Autodesk Inventor part; units mm, degrees
ref_plane "YZ Plane" through (0, 0, 0) normal (1, 0, 0) x (0, 1, 0)
ref_plane "XZ Plane" through (0, 0, 0) normal (0, 1, 0) x (-1, 0, 0)
ref_plane "XY Plane" through (0, 0, 0) normal (0, 0, 1) x (1, 0, 0)
sketch "Boceto1" plane through (0, 0, 0) normal (0, 0, 1) x (1, 0, 0)
  line L0 (-200, -200) -> (200, -200)
  line L1 (200, -200) -> (200, 200)
  line L2 (200, 200) -> (-200, 200)
  line L3 (-200, 200) -> (-200, -200)
  line L4 (-200, -200) -> (200, 200) construction
  line L5 (200, -200) -> (-200, 200) construction
  line L6 (-197.5, -197.5) -> (197.5, -197.5)
  line L7 (197.5, -197.5) -> (197.5, 197.5)
  line L8 (197.5, 197.5) -> (-197.5, 197.5)
  line L9 (-197.5, 197.5) -> (-197.5, -197.5)
  line L10 (-197.5, -197.5) -> (197.5, 197.5) construction
  line L11 (197.5, -197.5) -> (-197.5, 197.5) construction
  point P0 (0, 0)
  dimension "d0" = 400
  dimension "d1" = 400
  dimension "d2" = 395
  dimension "d3" = 395
extrude "Extrusión1" add sketch "Boceto1" along normal blind 5 contours L9 L8 L7 L6
extrude "Extrusión2" add sketch "Boceto1" along normal blind 400
properties part number "BOX"
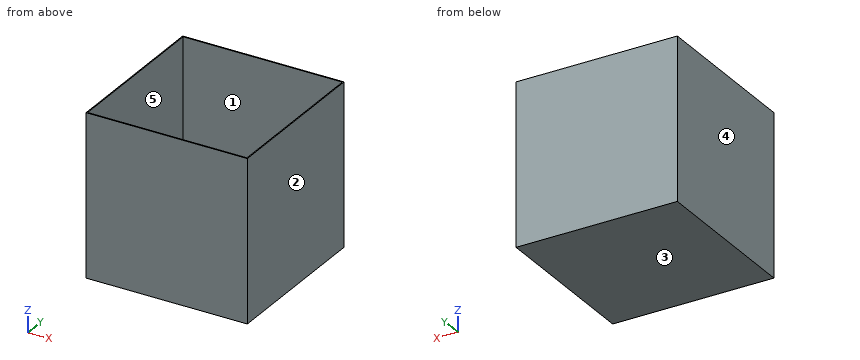
Work out the finished part from the listing and answer in its coordinate system (mm). Face numbers are marked on the shaded views. A direction names the side the tool comes from. Round coordinates to 2 decimals unless told otherwise and drop trailing zeros. Loops run counter-clockwise (first coordinate to the right, second up) from the corner with the lowest first, then second, coordinate; pieces in that order, holes last.
(1) This flat-tipped pin is pushed along its axis until it touches: P1, Ø4, axis at x = 49.5, y = 125.5, coming from the +Z side. Where does it stop, or does it pass through?
Computed values:
P1: stops at z = 5
(2) The part is cut by section B-B, the plane x = 53.5. Give the vertices of the cut face in (y, z).
Computed values:
outline: (-200, 0) - (200, 0) - (200, 400) - (197.5, 400) - (197.5, 5) - (-197.5, 5) - (-197.5, 400) - (-200, 400) - close
(3) For the marked faces 4 and 5, determine the directions among +Z, -Z, +X, -X, +Y, -Y from which every point of the face is accessible in a straight line to the end or side of a thin tool.
Computed values:
face 4: +Z, -Z, -X, +Y, -Y
face 5: +Z
(4) Find the intervals of material crossed by L1, parallel to X at y = 45.5, z = 270; L2, parallel to Z at x = -82, y = 148.5, in increasing order.
Computed values:
L1: x = -200 to -197.5, 197.5 to 200
L2: z = 0 to 5
(5) The mould has two halves that part along X. Classify the marked faces 1, 2 and 3: pulls with the +X half, pulls with the -X half, needs draft (parallel to the pull), parting line crosses it, or undercut.
Computed values:
face 1: undercut
face 2: pulls with the +X half
face 3: needs draft
(6) The part is cut by section A-A, the plane z = 233.5. Give the vertices of the cut face in (x, y), and give its area (4 significant figures).
Computed values:
outline: (-200, -200) - (200, -200) - (200, 200) - (-200, 200) - close; hole (-197.5, -197.5) - (197.5, -197.5) - (197.5, 197.5) - (-197.5, 197.5) - close
area: 3,975 mm2
